Can you work these out from the model? Positions are in its coordinate system, mm. A direction names the side the tool comes from. Coordinates: 2 decimals unless noted, no trailing zeros. Order: outer loops, then holes, each group sorted by start corner. A loop starts at its lowest first (then second) coordinate and runs counter-clockwise, first axis right, second up. Notation, with made-up numbers: (23.5, 51.25) -> (31.5, 51.25) arc R16 ccw to (31.5, 80.25) -> close; hole circle Ø3 at (87.5, 54). An arc over 180 degrees is marked (long way). Return JSON: item names as keys, results as strings. Group by question number.
1) For pin 1 (4.5 mm diameter, centred on x = 0, y = 100, fed in from +Z); pin 2 (2 mm diameter, centred on x = 0, y = 180, fed in from -Z), each with a flat end and sliding along its axis, tell me the tip position at first contact or that it passes through.
2) Thinking about a two-plate mould opening in Y: for faces 6 (the cylindrical face through (1.066, 186.614, 6.508)), 7 (the flat face through (0, 99, -7.1)), 8 (the flat face through (0.1, 0, -6.2)), 9 (the flat face through (0.1, 200, -6.2)), which applies, +Y half, -Y half, draft (parallel to the pull), parting line (faces both ways), or undercut?
3) If we section it at A-A, the plane z = 1.5: Please give me the cut outline in (x, y).
4) If we section it at C-C, the plane x = 0: Please give me the cut outline in (y, z), then the cut area to 3 significant figures.
5) If we section it at B-B, the plane y = 159: Please give me the cut outline in (x, z).
6) If I drill on probe 1 along Y at (x, z) = (0, -6.35); probe 2 along Y at (x, z) = (0, 6.7); probe 3 along Z at (x, y) = (-5.5, 120), over which ranges is the centre line in solid material (lowest first)? Write a range as from..to.
7) If we section it at D-D, the plane y = 20: Please give me the cut outline in (x, z), then the cut area to 3 significant figures.
8) For faces 1 (the cylindrical face through (0.496, 181.574, -6.508)), 2 (the flat face through (2, 99, 7.1)), 3 (the cylindrical face through (0.07, 101.65, 6.51)), 4 (the flat face through (7.1, 99, 0)), 5 (the flat face through (0, 99, -5.9)), which set-ups out of +Z, -Z, +X, -X, +Y, -Y let a thin tool reach every point of the face, with its end or its side?
Solid Edge part; units mm, degrees
sketch "Sketch1" plane through (0, 0, 0) normal (0, -1, 0) x (1, 0, 0)
  line L0 (-7.1, -7.1) -> (7.1, -7.1)
  line L1 (7.1, -7.1) -> (7.1, 7.1)
  line L2 (7.1, 7.1) -> (-7.1, 7.1)
  line L3 (-7.1, 7.1) -> (-7.1, -7.1)
  line L4 (-5.9, -5.9) -> (5.9, -5.9)
  line L5 (5.9, -5.9) -> (5.9, 5.9)
  line L6 (5.9, 5.9) -> (-5.9, 5.9)
  line L7 (-5.9, 5.9) -> (-5.9, -5.9)
extrude "Extrusionsausprägung_1" add sketch "Sketch1" against normal blind 200
hole "Bohrung_1" at (0, 100, 7.1) direction (0, 0, -1) diameter 3.3 end up to next
hole "Hole1" at (0, 10, 7.1) direction (0, 0, -1) diameter 3.3 end up to next
hole "Hole2" at (0, 190, 7.1) direction (0, 0, -1) diameter 3.3 end up to next
hole "Bohrung_4" at (0, 10, 7.1) direction (0, 0, -1) diameter 7.1 end up to next
hole "Hole3" at (0, 190, 7.1) direction (0, 0, -1) diameter 7.1 end up to next
hole "Bohrung_8" at (0, 20, -7.1) direction (0, 0, 1) diameter 3.3 end up to next
hole "Hole4" at (0, 180, -7.1) direction (0, 0, 1) diameter 3.3 end up to next
properties material "Aluminium, 2024-T4"
Result sheet:
{
 "1": {"pin 1": "stops at z = 7.1", "pin 2": "stops at z = 5.9"},
 "2": {"face 6": "undercut", "face 7": "draft", "face 8": "-Y half", "face 9": "+Y half"},
 "3": {"outline": "(-7.1, 0) -> (-5.9, 0) -> (-5.9, 200) -> (-7.1, 200) -> close; (5.9, 0) -> (7.1, 0) -> (7.1, 200) -> (5.9, 200) -> close"},
 "4": {"outline": "(0, -7.1) -> (18.35, -7.1) -> (18.35, -5.9) -> (0, -5.9) -> close; (0, 5.9) -> (6.45, 5.9) -> (6.45, 7.1) -> (0, 7.1) -> close; (13.55, 5.9) -> (98.35, 5.9) -> (98.35, 7.1) -> (13.55, 7.1) -> close; (21.65, -7.1) -> (178.35, -7.1) -> (178.35, -5.9) -> (21.65, -5.9) -> close; (101.65, 5.9) -> (186.45, 5.9) -> (186.45, 7.1) -> (101.65, 7.1) -> close; (181.65, -7.1) -> (200, -7.1) -> (200, -5.9) -> (181.65, -5.9) -> close; (193.55, 5.9) -> (200, 5.9) -> (200, 7.1) -> (193.55, 7.1) -> close", "area": "451 mm2"},
 "5": {"outline": "(-7.1, -7.1) -> (7.1, -7.1) -> (7.1, 7.1) -> (-7.1, 7.1) -> close; hole (-5.9, -5.9) -> (5.9, -5.9) -> (5.9, 5.9) -> (-5.9, 5.9) -> close"},
 "6": {"probe 1": "y = 0..18.35, 21.65..178.35, 181.65..200", "probe 2": "y = 0..6.45, 13.55..98.35, 101.65..186.45, 193.55..200", "probe 3": "z = -7.1..-5.9, 5.9..7.1"},
 "7": {"outline": "(-7.1, -7.1) -> (-1.65, -7.1) -> (-1.65, -5.9) -> (-5.9, -5.9) -> (-5.9, 5.9) -> (5.9, 5.9) -> (5.9, -5.9) -> (1.65, -5.9) -> (1.65, -7.1) -> (7.1, -7.1) -> (7.1, 7.1) -> (-7.1, 7.1) -> close", "area": "58.4 mm2"},
 "8": {"face 1": "-Z", "face 2": "+Z, +X, -X, +Y, -Y", "face 3": "+Z", "face 4": "+Z, -Z, +X, +Y, -Y", "face 5": "+Y, -Y"}
}
